from build123d import *

# Parameters (mm, degrees)
SKETCH1_W               = 80
SKETCH1_H               = 36
BOSS_EXTRUDE1_DEPTH     = 150
M2_5_TAPPED_HOLE1_D     = 2.05
M2_5_TAPPED_HOLE1_DEPTH = 3.35
M2_5_TAPPED_HOLE1_TIP   = 0.615882135
BOSS_EXTRUDE2_DEPTH     = 80
SKETCH7_W               = 20
SKETCH7_H               = 40
CUT_EXTRUDE4_DEPTH      = 80
SKETCH5_R               = 10.5
CUT_EXTRUDE5_DEPTH      = 80
SKETCH8_R               = 16
CUT_EXTRUDE6_DEPTH      = 7


with BuildPart() as part:
    # Sketch1 → Boss-Extrude1 (new body)
    with BuildSketch(Plane.XY):
        with Locations((40, 18)):
            Rectangle(SKETCH1_W, SKETCH1_H)
    extrude(amount=BOSS_EXTRUDE1_DEPTH)

    # M2.5 Tapped Hole1
    with Locations(Plane(origin=(25, 28, 150), x_dir=(1, 0, 0), z_dir=(0, 0, 1))):
        with Locations((0, 0), (30, 0), (30, -20), (0, -20)):
            Hole(M2_5_TAPPED_HOLE1_D / 2, depth=M2_5_TAPPED_HOLE1_DEPTH)
            with Locations((0, 0, -(M2_5_TAPPED_HOLE1_DEPTH + M2_5_TAPPED_HOLE1_TIP / 2))):  # 118° drill point
                Cone(0, M2_5_TAPPED_HOLE1_D / 2, M2_5_TAPPED_HOLE1_TIP, mode=Mode.SUBTRACT)

    # Sketch4 → Boss-Extrude2 (add)
    with BuildSketch(Plane.ZY):
        with BuildLine():
            Line((0, 36), (0, 0))
            ThreePointArc((0, 0), (-18, 18), (0, 36))
        make_face()
    extrude(amount=-BOSS_EXTRUDE2_DEPTH)

    # Sketch7 → Cut-Extrude4 (cut)
    with BuildSketch(Plane(origin=(0, 36, 0), x_dir=(1, 0, 0), z_dir=(0, 1, 0))):
        with Locations((10, -2)):
            Rectangle(SKETCH7_W, SKETCH7_H)
        with Locations((70, -2)):
            Rectangle(SKETCH7_W, SKETCH7_H)
    extrude(amount=-CUT_EXTRUDE4_DEPTH, mode=Mode.SUBTRACT)

    # Sketch5 → Cut-Extrude5 (cut)
    with BuildSketch(Plane.ZY):
        with Locations((0, 18)):
            Circle(SKETCH5_R)
    extrude(amount=-CUT_EXTRUDE5_DEPTH, mode=Mode.SUBTRACT)

    # Sketch8 → Cut-Extrude6 (cut)
    with BuildSketch(Plane.ZY.offset(-20)):
        with Locations((0, 18)):
            Circle(SKETCH8_R)
    cut_extrude6 = extrude(amount=-CUT_EXTRUDE6_DEPTH, mode=Mode.SUBTRACT)

    # Mirror1: Cut-Extrude6 across plane
    add(cut_extrude6.mirror(Plane.ZY.offset(-40)), mode=Mode.SUBTRACT)


solid = part.part
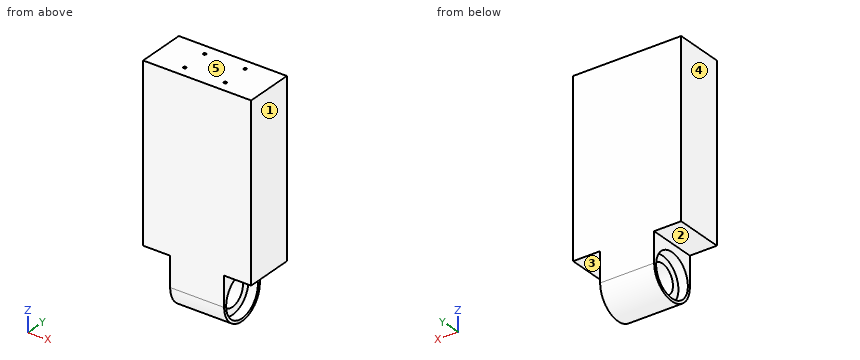
Source: CAD feature listing. Evaluate the final solid. Frame: model axes, mm. Face numbers are marked on the shaded views. A direction names the side the tool comes from. Round coordinates to 2 decimals unless told otherwise and drop trailing zeros. Loops run counter-clockwise (first coordinate to the right, second up) from the corner with the lowest first, then second, coordinate; pieces in that order, holes last. Notation, with made-up numbers: (45.5, 64) - (78.5, 64) arc R33 cw to (78.5, 92) - close; hole circle Ø10 at (44, 46). An arc over 180 degrees is marked (long way). Write item = value, one per line. Start each with the question number.
Item 1: Section query D-D on y = 31. Output: boundary loops of the cut face in (x, z).
Item 2: First-contact query: pin 1 Ø1.8 at (x, y) = (25, 28) entering from -Z; pin 2 Ø16 at (x, y) = (5.5, 24.5) entering from -Z; pin 3 Ø11 at (y, z) = (25.5, 0) entering from +X; pin 4 Ø12.5 at (y, z) = (18, 0) entering from +X. Flat tips, straight axial feed; report the tip coordinate or a pass-through.
Item 3: Section query B-B on x = 36.5. Output: boundary loops of the cut face in (y, z).
Item 4: Section query A-A on y = 18. Output: boundary loops of the cut face in (x, z), plus the area to 3 significant figures.
Item 5: Reachability of the marked faces 1 and 2 from +Z, -Z, +X, -X, +Y, -Y: full face, straight path, thin tool, end or side. Return the list, or none.
Item 6: Material intervals for line 1 (X direction, y = 8, z = 149.2) (3 decimals); line 2 (Y direction, x = 55, z = 147.6) (3 decimals); line 3 (Z direction, x = 76, y = 20), sorted ascending.
Item 7: Mould query, pull axis Z, two halves, no side actions, for the marked faces 3, 4 and 5. Classes: released by +Z, released by -Z, zero draft, split by the parting line, or undercut.
Item 8: Section query C-C on x = 75. Output: boundary loops of the cut face in (y, z).
Results list:
q1.outline = (0, 22) - (20, 22) - (20, 9.33) - (27, 9.33) - (27, -9.33) - (20, -9.33) - (20, -12.45) - (60, -12.45) - (60, -9.33) - (53, -9.33) - (53, 9.33) - (60, 9.33) - (60, 22) - (80, 22) - (80, 150) - (0, 150) - close
q2.pin_1 = -15.53
q2.pin_2 = 22
q2.pin_3 = 53
q2.pin_4 = through
q3.outline = (0, 0) arc R18 ccw to (36, 0) - (36, 150) - (0, 150) - close; hole circle Ø21 at (18, 0)
q4.outline = (0, 22) - (20, 22) - (20, 16) - (27, 16) - (27, 10.5) - (53, 10.5) - (53, 16) - (60, 16) - (60, 22) - (80, 22) - (80, 150) - (0, 150) - close; (20, -18) - (60, -18) - (60, -16) - (53, -16) - (53, -10.5) - (27, -10.5) - (27, -16) - (20, -16) - close
q4.area = 10,800 mm²
q5.face_1 = +Z, -Z, +X, +Y, -Y
q5.face_2 = -Z, -X, +Y, -Y
q6.line_1 = 0 to 23.975, 26.025 to 53.975, 56.025 to 80
q6.line_2 = 0 to 6.975, 9.025 to 26.975, 29.025 to 36
q6.line_3 = 22 to 150
q7.face_3 = released by -Z
q7.face_4 = zero draft
q7.face_5 = released by +Z
q8.outline = (0, 22) - (36, 22) - (36, 150) - (0, 150) - close
